from build123d import *

# Parameters (mm, degrees)
EXTRUDE_1_DEPTH             = 4
HOLE_WIZARD_M61_AT_2_COUNT  = 2
HOLE_WIZARD_M61_AT_2_PITCH  = 258
HOLE_WIZARD_M61_AT_3_COUNT  = 2
HOLE_WIZARD_M61_AT_3_PITCH  = 50
HOLE_WIZARD_M61_AT_4_COUNT  = 2
HOLE_WIZARD_M61_AT_4_PITCH  = 262.800304414
HOLE_WIZARD_M61_AT_5_COUNT  = 2
HOLE_WIZARD_M61_AT_5_PITCH  = 100
HOLE_WIZARD_M61_AT_6_COUNT  = 2
HOLE_WIZARD_M61_AT_6_PITCH  = 276.702005775
HOLE_WIZARD_M61_AT_7_COUNT  = 2
HOLE_WIZARD_M61_AT_7_PITCH  = 150
HOLE_WIZARD_M61_AT_8_COUNT  = 2
HOLE_WIZARD_M61_AT_8_PITCH  = 298.435922771
HOLE_WIZARD_M61_AT_9_COUNT  = 2
HOLE_WIZARD_M61_AT_9_PITCH  = 200
HOLE_WIZARD_M61_AT_10_COUNT = 2
HOLE_WIZARD_M61_AT_10_PITCH = 326.441418941
HOLE_WIZARD_M61_AT_11_COUNT = 2
HOLE_WIZARD_M61_AT_11_PITCH = 250
HOLE_WIZARD_M61_AT_12_COUNT = 2
HOLE_WIZARD_M61_AT_12_PITCH = 359.254784241
HOLE_WIZARD_M61_AT_13_COUNT = 2
HOLE_WIZARD_M61_AT_13_PITCH = 300
HOLE_WIZARD_M61_AT_14_COUNT = 2
HOLE_WIZARD_M61_AT_14_PITCH = 395.681690251


with BuildPart() as part:
    # Эскиз1 → Бобышка-Вытянуть1 (new body)
    with BuildSketch(Plane.XY):
        Polygon((0, 400), (-40, 400), (-40, 40), (0, 40), (0, 0), (218, 0), (218, 40), (258, 40), (258, 400), (218, 400), align=None)
    extrude(amount=EXTRUDE_1_DEPTH)

    # Эскиз2 → Зенковка для винта с потайной головкой и внутренним шестигранником M61 (revolve, cut)
    with BuildSketch(Plane(origin=(238, 70, 4), x_dir=(0, -1, 0), z_dir=(1, 0, 0))):
        Polygon((0, 0), (0, 4), (3.3, 4), (3.3, 3.555), (6.855, 0), align=None)
    hole_wizard_m61 = revolve(axis=Axis((238, 70, 10.35), (0, 0, -1)), mode=Mode.SUBTRACT)

    # Зенковка для винта с потайной головкой и внутренним шестигранником M61 at 2: Зенковка для винта с потайной головкой и внутренним шестигранником M61 ×2
    with Locations(*[(-i * HOLE_WIZARD_M61_AT_2_PITCH, 0, 0) for i in range(1, HOLE_WIZARD_M61_AT_2_COUNT)]):
        add(hole_wizard_m61, mode=Mode.SUBTRACT)

    # Зенковка для винта с потайной головкой и внутренним шестигранником M61 at 3: Зенковка для винта с потайной головкой и внутренним шестигранником M61 ×2
    with Locations(*[(0, i * HOLE_WIZARD_M61_AT_3_PITCH, 0) for i in range(1, HOLE_WIZARD_M61_AT_3_COUNT)]):
        add(hole_wizard_m61, mode=Mode.SUBTRACT)

    # Зенковка для винта с потайной головкой и внутренним шестигранником M61 at 4: Зенковка для винта с потайной головкой и внутренним шестигранником M61 ×2
    with Locations(*[Vector(-0.9817340226278134, 0.19025853151701805, 0) * (i * HOLE_WIZARD_M61_AT_4_PITCH) for i in range(1, HOLE_WIZARD_M61_AT_4_COUNT)]):
        add(hole_wizard_m61, mode=Mode.SUBTRACT)

    # Зенковка для винта с потайной головкой и внутренним шестигранником M61 at 5: Зенковка для винта с потайной головкой и внутренним шестигранником M61 ×2
    with Locations(*[(0, i * HOLE_WIZARD_M61_AT_5_PITCH, 0) for i in range(1, HOLE_WIZARD_M61_AT_5_COUNT)]):
        add(hole_wizard_m61, mode=Mode.SUBTRACT)

    # Зенковка для винта с потайной головкой и внутренним шестигранником M61 at 6: Зенковка для винта с потайной головкой и внутренним шестигранником M61 ×2
    with Locations(*[Vector(-0.9324110220206997, 0.36139962093825506, 0) * (i * HOLE_WIZARD_M61_AT_6_PITCH) for i in range(1, HOLE_WIZARD_M61_AT_6_COUNT)]):
        add(hole_wizard_m61, mode=Mode.SUBTRACT)

    # Зенковка для винта с потайной головкой и внутренним шестигранником M61 at 7: Зенковка для винта с потайной головкой и внутренним шестигранником M61 ×2
    with Locations(*[(0, i * HOLE_WIZARD_M61_AT_7_PITCH, 0) for i in range(1, HOLE_WIZARD_M61_AT_7_COUNT)]):
        add(hole_wizard_m61, mode=Mode.SUBTRACT)

    # Зенковка для винта с потайной головкой и внутренним шестигранником M61 at 8: Зенковка для винта с потайной головкой и внутренним шестигранником M61 ×2
    with Locations(*[Vector(-0.8645071866841932, 0.5026204573745298, 0) * (i * HOLE_WIZARD_M61_AT_8_PITCH) for i in range(1, HOLE_WIZARD_M61_AT_8_COUNT)]):
        add(hole_wizard_m61, mode=Mode.SUBTRACT)

    # Зенковка для винта с потайной головкой и внутренним шестигранником M61 at 9: Зенковка для винта с потайной головкой и внутренним шестигранником M61 ×2
    with Locations(*[(0, i * HOLE_WIZARD_M61_AT_9_PITCH, 0) for i in range(1, HOLE_WIZARD_M61_AT_9_COUNT)]):
        add(hole_wizard_m61, mode=Mode.SUBTRACT)

    # Зенковка для винта с потайной головкой и внутренним шестигранником M61 at 10: Зенковка для винта с потайной головкой и внутренним шестигранником M61 ×2
    with Locations(*[Vector(-0.7903408851647249, 0.61266735284087, 0) * (i * HOLE_WIZARD_M61_AT_10_PITCH) for i in range(1, HOLE_WIZARD_M61_AT_10_COUNT)]):
        add(hole_wizard_m61, mode=Mode.SUBTRACT)

    # Зенковка для винта с потайной головкой и внутренним шестигранником M61 at 11: Зенковка для винта с потайной головкой и внутренним шестигранником M61 ×2
    with Locations(*[(0, i * HOLE_WIZARD_M61_AT_11_PITCH, 0) for i in range(1, HOLE_WIZARD_M61_AT_11_COUNT)]):
        add(hole_wizard_m61, mode=Mode.SUBTRACT)

    # Зенковка для винта с потайной головкой и внутренним шестигранником M61 at 12: Зенковка для винта с потайной головкой и внутренним шестигранником M61 ×2
    with Locations(*[Vector(-0.7181532753840043, 0.6958849567674433, 0) * (i * HOLE_WIZARD_M61_AT_12_PITCH) for i in range(1, HOLE_WIZARD_M61_AT_12_COUNT)]):
        add(hole_wizard_m61, mode=Mode.SUBTRACT)

    # Зенковка для винта с потайной головкой и внутренним шестигранником M61 at 13: Зенковка для винта с потайной головкой и внутренним шестигранником M61 ×2
    with Locations(*[(0, i * HOLE_WIZARD_M61_AT_13_PITCH, 0) for i in range(1, HOLE_WIZARD_M61_AT_13_COUNT)]):
        add(hole_wizard_m61, mode=Mode.SUBTRACT)

    # Зенковка для винта с потайной головкой и внутренним шестигранником M61 at 14: Зенковка для винта с потайной головкой и внутренним шестигранником M61 ×2
    with Locations(*[Vector(-0.6520392688280492, 0.7581851963116815, 0) * (i * HOLE_WIZARD_M61_AT_14_PITCH) for i in range(1, HOLE_WIZARD_M61_AT_14_COUNT)]):
        add(hole_wizard_m61, mode=Mode.SUBTRACT)


solid = part.part
Source: CAD feature listing. Evaluate the final solid. Frame: model axes, mm. Round coordinates to 2 decimals unless told otherwise and drop trailing zeros.
Q1. Mould query, pull axis Y, two halves, no side actions, for faces 1 (the face through (107, 203, 4)), 2 (the face through (-21.06, 116.64, 0.67)). Classes: pulls with the +Y half, pulls with the -Y half, needs draft (parallel to the pull), parting line crosses it, or undercut.
Q2. Ray query, line 1 (X direction, y = 120, z = 0.3); line 2 (X direction, y = 217, z = 1.25); line 3 (Z direction, x = 239.5, y = 374.5). Return the intervals inside material, ascending.
Q3. Section A-A, the plane z = 2.3. State how many separate pieces and enclosed holes the cut face has, plus the area to 3 significant figures.
Solutions:
1. face 1: needs draft
1. face 2: undercut
2. line 1: x = -40 to -23.3, -16.7 to 234.7, 241.3 to 258
2. line 2: x = -40 to -22.8, -17.2 to 235.2, 240.8 to 258
2. line 3: z = 0 to 1.89
3. separate pieces: 1
3. enclosed holes: 14
3. area: 115,000 mm2
